```python
from build123d import *

# Parameters (mm, degrees)
SKETCH1_R           = 12.5
SKETCH1_R_2         = 4.75
BOSS_EXTRUDE1_DEPTH = 5
SKETCH1_3_R         = 4.75
SKETCH1_3_W         = 5.6
SKETCH1_3_H         = 4.6
BOSS_EXTRUDE2_DEPTH = 13
SKETCH1_4_W         = 5.6
SKETCH1_4_H         = 4.6
BOSS_EXTRUDE3_DEPTH = 19.5
SKETCH2_R           = 3.5
CUT_EXTRUDE2_DEPTH  = 3
SKETCH2_3_R         = 3.5
CUT_EXTRUDE3_DEPTH  = 4


with BuildPart() as part:
    # Sketch1 → Boss-Extrude1 (new body)
    with BuildSketch(Plane(origin=(0, 0, 0), x_dir=(1, 0, 0), z_dir=(0, 1, 0))):
        with Locations(Location((0, 0, 0), (0, 0, 270))):
            Circle(SKETCH1_R)
        with Locations(Location((0, 0, 0), (0, 0, 270))):
            Circle(SKETCH1_R_2, mode=Mode.SUBTRACT)
    extrude(amount=BOSS_EXTRUDE1_DEPTH)

    # Sketch1_3 → Boss-Extrude2 (add)
    with BuildSketch(Plane(origin=(0, 0, 0), x_dir=(1, 0, 0), z_dir=(0, 1, 0))):
        with Locations(Location((0, 0, 0), (0, 0, 270))):
            Circle(SKETCH1_3_R)
        Rectangle(SKETCH1_3_W, SKETCH1_3_H, mode=Mode.SUBTRACT)
    extrude(amount=BOSS_EXTRUDE2_DEPTH)

    # Sketch1_4 → Boss-Extrude3 (add)
    with BuildSketch(Plane(origin=(0, 0, 0), x_dir=(1, 0, 0), z_dir=(0, 1, 0))):
        Rectangle(SKETCH1_4_W, SKETCH1_4_H)
    extrude(amount=BOSS_EXTRUDE3_DEPTH)

    # Sketch2 → Cut-Extrude2 (cut)
    with BuildSketch(Plane(origin=(0, 0, 0), x_dir=(1, 0, 0), z_dir=(0, 1, 0))):
        Circle(SKETCH2_R)
        with BuildLine():
            Line((-0.288199979, -3.488114214), (-12.247448714, -2.5))
            ThreePointArc((-12.247448714, -2.5), (-12.5, 0), (-12.247448714, 2.5))
            Line((-12.247448714, 2.5), (-0.288199979, 3.488114214))
            ThreePointArc((-0.288199979, 3.488114214), (3.5, 0), (-0.288199979, -3.488114214))
        make_face()
    extrude(amount=CUT_EXTRUDE2_DEPTH, mode=Mode.SUBTRACT)

    # Sketch2_3 → Cut-Extrude3 (cut)
    with BuildSketch(Plane(origin=(0, 0, 0), x_dir=(1, 0, 0), z_dir=(0, 1, 0))):
        with Locations(Location((0, 0, 0), (0, 0, 94.723245675))):
            Circle(SKETCH2_3_R)
    extrude(amount=CUT_EXTRUDE3_DEPTH, mode=Mode.SUBTRACT)


solid = part.part
```
Here's how the part is built. I have some questions about the finished solid (model axes, mm). A direction names the side the tool comes from. Coordinates: 2 decimals unless noted, no trailing zeros. Order: outer loops, then holes, each group sorted by start corner. A loop starts at its lowest first (then second) coordinate and runs counter-clockwise, first axis right, second up.
1) Imagine slicing it at B-B on x = -9.25. List the corners of the cut face in (y, z) for me, and give its area (3 significant figures).
2) Imagine slicing it at D-D on z = -3. List the corners of the cut face in (x, y) for me, and give its area (3 significant figures).
3) Imagine slicing it at A-A on z = 0. List the corners of the cut face in (x, y) for me, and give its area (3 significant figures).
4) We'd pull the mould along X, two halves only. Please class faces 1 (the face through (2.8, 16, 0)), 2 (the face through (-6.352, 1.479, -2.987)), 3 (the face through (0, 16, 2.3)): +X half, -X half, draft (parallel to the pull), parting line (faces both ways), or undercut.
5) Which directions (+Z, -Z, +X, -X, +Y, -Y) give clear straight access to the entire face, cutting with the end or side of a thin tool? Please do faces 4 (the face through (-2.8, 16, 0)), 5 (the face through (0, 16, -2.3)), 6 (the face through (-5, 5, 0)), 7 (the face through (0, 4, 0)), 8 (the face through (0, 19.5, 0)).
6) Will these pins go through, and if not, where does the flat tip stop? pin 1 (3.5 mm diameter, centred on x = -5, z = -1, fed in from -Y); pin 2 (6 mm diameter, centred on x = -1, y = 17.5, fed in from +Z); pin 3 (1.7 mm diameter, centred on x = 1, y = 15, fed in from -Z); pin 4 (1 mm diameter, centred on y = 14.5, z = 6.5, fed in from +X).
7) I need wall thicknesses on line 1 (Z direction, x = 0, y = 1.9); line 2 (X direction, y = 4.5, z = 0.25). Which ranges of each line are inside material? Lowest first, please.
8) Imagine slicing it at C-C on y = 2.5. List the corners of the cut face in (x, z) for me.
Response values:
1. outline: (0, -8.41) - (5, -8.41) - (5, 8.41) - (0, 8.41) - (0, 2.75) - (3, 2.75) - (3, -2.75) - (0, -2.75) - close
1. area: 67.6 mm2
2. outline: (-12.13, 0) - (-6.2, 0) - (-6.2, 3) - (-1.8, 3) - (-1.8, 4) - (1.8, 4) - (1.8, 0) - (12.13, 0) - (12.13, 5) - (3.68, 5) - (3.68, 13) - (-3.68, 13) - (-3.68, 5) - (-12.13, 5) - close
2. area: 153 mm2
3. outline: (-12.5, 3) - (-3.5, 3) - (-3.5, 4) - (3.5, 4) - (3.5, 0) - (12.5, 0) - (12.5, 5) - (4.75, 5) - (4.75, 13) - (2.8, 13) - (2.8, 19.5) - (-2.8, 19.5) - (-2.8, 13) - (-4.75, 13) - (-4.75, 5) - (-12.5, 5) - close
3. area: 182 mm2
4. face 1: +X half
4. face 2: undercut
4. face 3: draft
5. face 4: +Z, -Z, -X, +Y
5. face 5: -Z, +X, -X, +Y
5. face 6: +Y
5. face 7: -Y
5. face 8: +Z, -Z, +X, -X, +Y
6. pin 1: stops at y = 3
6. pin 2: stops at z = 2.3
6. pin 3: stops at z = -2.3
6. pin 4: passes through
7. line 1: z = -12.5 to -3.5, 3.5 to 12.5
7. line 2: x = -12.5 to 12.5
8. outline: (-12.25, -2.5) arc R12.5 ccw (long way) to (-12.25, 2.5) - (-0.29, 3.49) arc R3.5 cw (long way) to (-0.29, -3.49) - close
